```python
from build123d import *

# Parameters (mm, degrees)
SKETCH1_R           = 2.5
BOSS_EXTRUDE1_DEPTH = 2
SKETCH2_R           = 1
BOSS_EXTRUDE2_DEPTH = 12
SKETCH3_R           = 2.5
BOSS_EXTRUDE3_DEPTH = 2
FILLET1_R           = 0.2


with BuildPart() as part:
    # Sketch1 → Boss-Extrude1 (new body)
    with BuildSketch(Plane(origin=(0, 0, 0), x_dir=(1, 0, 0), z_dir=(0, 1, 0))):
        Circle(SKETCH1_R)
    extrude(amount=-BOSS_EXTRUDE1_DEPTH)

    # Sketch2 → Boss-Extrude2 (add)
    with BuildSketch(Plane.XZ.offset(2)):
        Circle(SKETCH2_R)
    extrude(amount=BOSS_EXTRUDE2_DEPTH)

    # Sketch3 → Boss-Extrude3 (add)
    with BuildSketch(Plane.XZ.offset(14)):
        Circle(SKETCH3_R)
    extrude(amount=BOSS_EXTRUDE3_DEPTH)

    # Fillet1
    fillet1_edges = [part.edges().sort_by_distance(p)[0] for p in [
        (-2.5, 0, 0),
        (-2.5, -2, 0),
        (-2.5, -14, 0),
        (-2.5, -16, 0),
    ]]
    fillet(fillet1_edges, radius=FILLET1_R)


solid = part.part
```
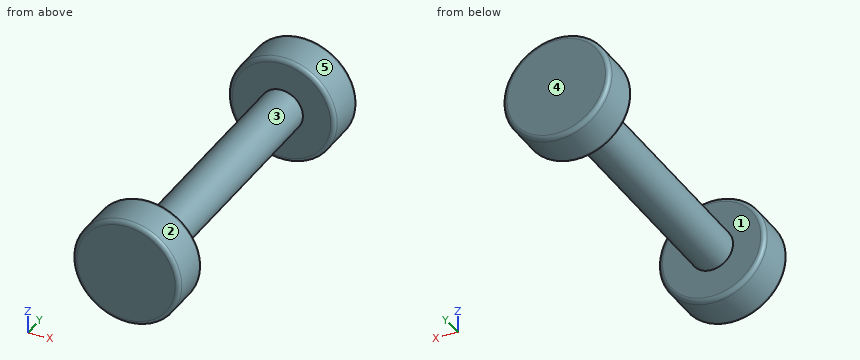
Part model, mm, in its own coordinate system. Face numbers are marked on the shaded views. A direction names the side the tool comes from. Round coordinates to 2 decimals unless told otherwise and drop trailing zeros. Write each loop counter-clockwise with the first axis right and the second up, starting at its lowest first coordinate (ties: lowest second). Pieces come first, ordered by that corner, then holes.
Item 1: Cut at A-A, the plane z = 0. Give the cut face in (x, y), plus the area to 3 significant figures.
Results:
outline: (-2.5, -15.8) arc R0.2 ccw to (-2.3, -16) - (2.3, -16) arc R0.2 ccw to (2.5, -15.8) - (2.5, -14.2) arc R0.2 ccw to (2.3, -14) - (1, -14) - (1, -2) - (2.3, -2) arc R0.2 ccw to (2.5, -1.8) - (2.5, -0.2) arc R0.2 ccw to (2.3, 0) - (-2.3, 0) arc R0.2 ccw to (-2.5, -0.2) - (-2.5, -1.8) arc R0.2 ccw to (-2.3, -2) - (-1, -2) - (-1, -14) - (-2.3, -14) arc R0.2 ccw to (-2.5, -14.2) - close
area: 43.9 mm2
Item 2: Probe L1, parallel to Y at x = 0.55, z = -1.8; L2, parallel to X at y = -11.75, z = 0.15; L3, parallel to Z at x = -0.3, y = -6.75. List the from-to ranges inside material, lowest first.
Results:
L1: y = -16 to -14, -2 to 0
L2: x = -0.99 to 0.99
L3: z = -0.95 to 0.95
Item 3: Two-plate mould, pull along Y, no slides. Class the marked faces 3, 4 and 5: +Y half, -Y half, draft (parallel to the pull), parting line (faces both ways), or undercut.
Results:
face 3: undercut
face 4: +Y half
face 5: draft
Item 4: Cut at B-B, the plane x = 0. Give the cut face in (y, z).
Results:
outline: (-16, -2.3) arc R0.2 ccw to (-15.8, -2.5) - (-14.2, -2.5) arc R0.2 ccw to (-14, -2.3) - (-14, -1) - (-2, -1) - (-2, -2.3) arc R0.2 ccw to (-1.8, -2.5) - (-0.2, -2.5) arc R0.2 ccw to (0, -2.3) - (0, 2.3) arc R0.2 ccw to (-0.2, 2.5) - (-1.8, 2.5) arc R0.2 ccw to (-2, 2.3) - (-2, 1) - (-14, 1) - (-14, 2.3) arc R0.2 ccw to (-14.2, 2.5) - (-15.8, 2.5) arc R0.2 ccw to (-16, 2.3) - close
Item 5: Cut at C-C, the plane y = -13.75. Give the cut face in (x, z).
Results:
outline: circle Ø2 at (0, 0)
Item 6: Drop flat-ended pins along their axis: pin 1 Ø1.5 at (y, z) = (-7.5, 0.5) entering from -X; pin 2 Ø1 at (x, z) = (0.5, 1) entering from +Y; pin 3 Ø2 at (x, y) = (-1, -11.5) entering from +Z; pin 4 Ø2 at (y, z) = (-12.5, -0.5) entering from +X. Give the stop position or say it passes through.
Results:
pin 1: stops at x = -1
pin 2: stops at y = 0
pin 3: stops at z = 1
pin 4: stops at x = 1
Item 7: Which spindle directions (+Z, -Z, +X, -X, +Y, -Y) get a long thin tool onto all of the face, cutting with end or side? Do the marked faces 1 and 2. Say none if no direction does.
Results:
face 1: none
face 2: +Y, -Y
